```python
from build123d import *

# Parameters (mm, degrees)
SKETCH1_W                                       = 140
SKETCH1_H                                       = 220
BOSS_EXTRUDE1_DEPTH                             = 5
CUT_EXTRUDE1_DEPTH                              = 5
CHAMFER3_SIZE                                   = 15
F_4_0_4_DIAMETER_HOLE3_D                        = 4
F_4_0_4_DIAMETER_HOLE3_DEPTH                    = 5
F_4_0_4_DIAMETER_HOLE3_TIP                      = 1.201721238
CSK_FOR_M3_FLAT_HEAD_MACHINE_SCREW4_D           = 3.4
CSK_FOR_M3_FLAT_HEAD_MACHINE_SCREW4_DEPTH       = 5
CSK_FOR_M3_FLAT_HEAD_MACHINE_SCREW4_CSINK_D     = 6.3
CSK_FOR_M3_FLAT_HEAD_MACHINE_SCREW4_CSINK_ANGLE = 90
CSK_FOR_M3_FLAT_HEAD_MACHINE_SCREW4_TIP         = 1.021463052
SKETCH18_W                                      = 81.237331022
SKETCH18_H                                      = 9.628563132
CUT_EXTRUDE2_DEPTH                              = 5
CUT_EXTRUDE8_DEPTH                              = 10
SKETCH35_W                                      = 65
SKETCH35_H                                      = 45
CUT_EXTRUDE9_DEPTH                              = 131.479883507
FILLET1_R                                       = 2
CUT_EXTRUDE10_DEPTH                             = 131.479883507
SKETCH38_W                                      = 36
SKETCH38_H                                      = 20
CUT_EXTRUDE14_DEPTH                             = 131.479883507
SKETCH39_R                                      = 7
CUT_EXTRUDE15_DEPTH                             = 131.479883507
CSK_FOR_M3_FLAT_HEAD_MACHINE_SCREW3_D           = 3.4
CSK_FOR_M3_FLAT_HEAD_MACHINE_SCREW3_DEPTH       = 10
CSK_FOR_M3_FLAT_HEAD_MACHINE_SCREW3_CSINK_D     = 6.3
CSK_FOR_M3_FLAT_HEAD_MACHINE_SCREW3_CSINK_ANGLE = 90
CSK_FOR_M3_FLAT_HEAD_MACHINE_SCREW3_TIP         = 1.021463052
BOSS_EXTRUDE2_START                             = -3
SKETCH42_R                                      = 7
SKETCH42_R_2                                    = 4.25
BOSS_EXTRUDE2_DEPTH                             = 3
BOSS_EXTRUDE3_START                             = 8
SKETCH43_R                                      = 9
SKETCH43_R_2                                    = 7
BOSS_EXTRUDE3_DEPTH                             = 8
F_4_0MM_DOWEL_HOLE1_AT_2_COUNT                  = 2
F_4_0MM_DOWEL_HOLE1_AT_2_PITCH                  = 108.54146673
CUT_EXTRUDE16_DEPTH                             = 2
BOSS_EXTRUDE4_DEPTH                             = 5
CSK_FOR_M3_FLAT_HEAD_MACHINE_SCREW2_D           = 3.4
CSK_FOR_M3_FLAT_HEAD_MACHINE_SCREW2_DEPTH       = 5
CSK_FOR_M3_FLAT_HEAD_MACHINE_SCREW2_CSINK_D     = 6.3
CSK_FOR_M3_FLAT_HEAD_MACHINE_SCREW2_CSINK_ANGLE = 90
CSK_FOR_M3_FLAT_HEAD_MACHINE_SCREW2_TIP         = 1.021463052
FILLET3_R                                       = 2


with BuildPart() as part:
    # Sketch1 → Boss-Extrude1 (new body)
    with BuildSketch(Plane(origin=(0, 0, 0), x_dir=(1, 0, 0), z_dir=(0, 1, 0))):
        Rectangle(SKETCH1_W, SKETCH1_H)
    extrude(amount=BOSS_EXTRUDE1_DEPTH)

    # Sketch8 → Cut-Extrude1 (cut)
    with BuildSketch(Plane(origin=(0, 5, 0), x_dir=(1, 0, 0), z_dir=(0, 1, 0))):
        Polygon((-70, 110), (-32.5, 110), (-32.5, 44.951905284), (-70, -20), align=None)
        Polygon((70, 110), (70, -20), (32.5, 44.951905284), (32.5, 110), align=None)
    extrude(amount=-CUT_EXTRUDE1_DEPTH, mode=Mode.SUBTRACT)

    # Chamfer3
    chamfer3_edges = [part.edges().sort_by_distance(p)[0] for p in [
        (70, 2.5, 110),
        (-70, 2.5, 110),
    ]]
    chamfer(chamfer3_edges, length=CHAMFER3_SIZE)

    # Ø4.0 (4) Diameter Hole3
    with Locations(Plane(origin=(0, 5, 0), x_dir=(1, 0, 0), z_dir=(0, 1, 0))):
        with Locations((-27, 78), (-27, 63), (-60.732233047, -90.125631329), (-50.125631329, -100.732233047), (50.125631329, -100.732233047), (60.732233047, -90.125631329), (27, 63), (27, 78)):
            Hole(F_4_0_4_DIAMETER_HOLE3_D / 2, depth=F_4_0_4_DIAMETER_HOLE3_DEPTH)
            with Locations((0, 0, -(F_4_0_4_DIAMETER_HOLE3_DEPTH + F_4_0_4_DIAMETER_HOLE3_TIP / 2))):  # 118° drill point
                Cone(0, F_4_0_4_DIAMETER_HOLE3_D / 2, F_4_0_4_DIAMETER_HOLE3_TIP, mode=Mode.SUBTRACT)

    # CSK for M3 Flat Head Machine Screw4
    with Locations(Plane.XZ):
        with Locations((37.5, -25), (-37.5, -25), (-25, -100), (25, -100)):
            CounterSinkHole(CSK_FOR_M3_FLAT_HEAD_MACHINE_SCREW4_D / 2, CSK_FOR_M3_FLAT_HEAD_MACHINE_SCREW4_CSINK_D / 2, depth=CSK_FOR_M3_FLAT_HEAD_MACHINE_SCREW4_DEPTH, counter_sink_angle=CSK_FOR_M3_FLAT_HEAD_MACHINE_SCREW4_CSINK_ANGLE)
            with Locations((0, 0, -(CSK_FOR_M3_FLAT_HEAD_MACHINE_SCREW4_DEPTH + CSK_FOR_M3_FLAT_HEAD_MACHINE_SCREW4_TIP / 2))):  # 118° drill point
                Cone(0, CSK_FOR_M3_FLAT_HEAD_MACHINE_SCREW4_D / 2, CSK_FOR_M3_FLAT_HEAD_MACHINE_SCREW4_TIP, mode=Mode.SUBTRACT)

    # Sketch18 → Cut-Extrude2 (cut)
    with BuildSketch(Plane(origin=(0, 5, 0), x_dir=(1, 0, 0), z_dir=(0, 1, 0))):
        with Locations((-5.815131093, 109.814281566)):
            Rectangle(SKETCH18_W, SKETCH18_H)
    extrude(amount=-CUT_EXTRUDE2_DEPTH, mode=Mode.SUBTRACT)

    # Sketch34 → Cut-Extrude8 (cut)
    with BuildSketch(Plane(origin=(0, 5, 0), x_dir=(1, 0, 0), z_dir=(0, 1, 0))):
        Polygon((-70, -20), (-60, -2.679491924), (-60, -72.679491924), (-70, -90), align=None)
        Polygon((70, -90), (70, -20), (60, -2.679491924), (60, -72.679491924), align=None)
    extrude(amount=-CUT_EXTRUDE8_DEPTH, mode=Mode.SUBTRACT)

    # Sketch35 → Cut-Extrude9 (cut, through all)
    with BuildSketch(Plane(origin=(0, 5, 0), x_dir=(1, 0, 0), z_dir=(0, 1, 0))):
        with Locations((2, -36)):
            Rectangle(SKETCH35_W, SKETCH35_H)
    extrude(amount=-CUT_EXTRUDE9_DEPTH, mode=Mode.SUBTRACT)

    # Fillet1
    fillet1_edges = [part.edges().sort_by_distance(p)[0] for p in [
        (34.5, 2.5, 13.5),
        (34.5, 2.5, 58.5),
        (-30.5, 2.5, 58.5),
        (-30.5, 2.5, 13.5),
    ]]
    fillet(fillet1_edges, radius=FILLET1_R)

    # Sketch36 → Cut-Extrude10 (cut, through all)
    with BuildSketch(Plane(origin=(0, 5, 0), x_dir=(1, 0, 0), z_dir=(0, 1, 0))):
        Polygon((-47.5, -110), (-37.5, -100), (37.5, -100), (47.5, -110), align=None)
    extrude(amount=-CUT_EXTRUDE10_DEPTH, mode=Mode.SUBTRACT)

    # Sketch38 → Cut-Extrude14 (cut, through all)
    with BuildSketch(Plane.XZ):
        with Locations((0, -95)):
            Rectangle(SKETCH38_W, SKETCH38_H)
    extrude(amount=-CUT_EXTRUDE14_DEPTH, mode=Mode.SUBTRACT)

    # Sketch39 → Cut-Extrude15 (cut, through all)
    with BuildSketch(Plane.XZ):
        with Locations(Location((-47.5, 30, 0), (0, 0, 270))):
            Circle(SKETCH39_R)
        with Locations(Location((47.5, 30, 0), (0, 0, 90))):
            Circle(SKETCH39_R)
    extrude(amount=-CUT_EXTRUDE15_DEPTH, mode=Mode.SUBTRACT)

    # CSK for M3 Flat Head Machine Screw3
    with Locations(Plane(origin=(0, 0, 0), x_dir=(-1, 0, 0), z_dir=(0, -1, 0))):
        with Locations((-58, -82), (58, -82)):
            CounterSinkHole(CSK_FOR_M3_FLAT_HEAD_MACHINE_SCREW3_D / 2, CSK_FOR_M3_FLAT_HEAD_MACHINE_SCREW3_CSINK_D / 2, depth=CSK_FOR_M3_FLAT_HEAD_MACHINE_SCREW3_DEPTH, counter_sink_angle=CSK_FOR_M3_FLAT_HEAD_MACHINE_SCREW3_CSINK_ANGLE)
            with Locations((0, 0, -(CSK_FOR_M3_FLAT_HEAD_MACHINE_SCREW3_DEPTH + CSK_FOR_M3_FLAT_HEAD_MACHINE_SCREW3_TIP / 2))):  # 118° drill point
                Cone(0, CSK_FOR_M3_FLAT_HEAD_MACHINE_SCREW3_D / 2, CSK_FOR_M3_FLAT_HEAD_MACHINE_SCREW3_TIP, mode=Mode.SUBTRACT)

    # Sketch42 → Boss-Extrude2 (add)
    # profile 1 of 2: a face of its own
    with BuildSketch(Plane(origin=(0, 5, 0), x_dir=(1, 0, 0), z_dir=(0, 1, 0)).offset(BOSS_EXTRUDE2_START)):
        with Locations(Location((-47.5, -30, 0), (0, 0, 90))):
            Circle(SKETCH42_R)
        with Locations(Location((-47.5, -30, 0), (0, 0, 270))):
            Circle(SKETCH42_R_2, mode=Mode.SUBTRACT)
    # profile 2 of 2: a face of its own
    with BuildSketch(Plane(origin=(0, 5, 0), x_dir=(1, 0, 0), z_dir=(0, 1, 0)).offset(BOSS_EXTRUDE2_START)):
        with Locations(Location((47.5, -30, 0), (0, 0, 90))):
            Circle(SKETCH42_R)
        with Locations(Location((47.5, -30, 0), (0, 0, 90))):
            Circle(SKETCH42_R_2, mode=Mode.SUBTRACT)
    extrude(amount=BOSS_EXTRUDE2_DEPTH)

    # Sketch43 → Boss-Extrude3 (add)
    # profile 1 of 2: a face of its own
    with BuildSketch(Plane.XZ.offset(BOSS_EXTRUDE3_START)):
        with Locations(Location((-47.5, 30, 0), (0, 0, 90))):
            Circle(SKETCH43_R)
        with Locations(Location((-47.5, 30, 0), (0, 0, 270))):
            Circle(SKETCH43_R_2, mode=Mode.SUBTRACT)
    # profile 2 of 2: a face of its own
    with BuildSketch(Plane.XZ.offset(BOSS_EXTRUDE3_START)):
        with Locations(Location((47.5, 30, 0), (0, 0, 90))):
            Circle(SKETCH43_R)
        with Locations(Location((47.5, 30, 0), (0, 0, 270))):
            Circle(SKETCH43_R_2, mode=Mode.SUBTRACT)
    extrude(amount=-BOSS_EXTRUDE3_DEPTH)

    # Sketch46 → Ø4.0mm Dowel Hole1 (revolve, cut)
    with BuildSketch(Plane(origin=(-54.5, 5, 54), x_dir=(0, 0, 1), z_dir=(1, 0, 0))):
        Polygon((0, 0), (0, 6.201721238), (2, 5), (2, 0), align=None)
    f_4_0mm_dowel_hole1 = revolve(axis=Axis((-54.5, 11.35, 54), (0, -1, 0)), mode=Mode.SUBTRACT)

    # Ø4.0mm Dowel Hole1 at 2: Ø4.0mm Dowel Hole1 ×2
    with Locations(*[Vector(0.2533593918376833, 0, -0.9673722233802454) * (i * F_4_0MM_DOWEL_HOLE1_AT_2_PITCH) for i in range(1, F_4_0MM_DOWEL_HOLE1_AT_2_COUNT)]):
        add(f_4_0mm_dowel_hole1, mode=Mode.SUBTRACT)

    # Mirror1: Ø4.0mm Dowel Hole1 across plane
    add(f_4_0mm_dowel_hole1.mirror(Plane(origin=(0, 0, 0), x_dir=(0, 0, 1), z_dir=(1, 0, 0))), mode=Mode.SUBTRACT)

    # Mirror1 copy 1 sketch → Mirror1 copy 1 (revolve, cut)
    with BuildSketch(Plane(origin=(27, 5, -51), x_dir=(0, 0, 1), z_dir=(-1, 0, 0))):
        Polygon((0, 0), (0, -6.201721238), (2, -5), (2, 0), align=None)
    revolve(axis=Axis((27, 11.35, -51), (0, 1, 0)), mode=Mode.SUBTRACT)

    # Sketch47 → Cut-Extrude16 (cut)
    with BuildSketch(Plane(origin=(0, 5, 0), x_dir=(1, 0, 0), z_dir=(0, 1, 0))):
        Polygon((29.8, 49.383419246), (29.8, 52.616580754), (27, 54.233161507), (24.2, 52.616580754), (24.2, 49.383419246), (27, 47.766838493), align=None)
        Polygon((57.3, -55.616580754), (57.3, -52.383419246), (54.5, -50.766838493), (51.7, -52.383419246), (51.7, -55.616580754), (54.5, -57.233161507), align=None)
        Polygon((-54.5, -57.233161507), (-57.3, -55.616580754), (-57.3, -52.383419246), (-54.5, -50.766838493), (-51.7, -52.383419246), (-51.7, -55.616580754), align=None)
        Polygon((-27, 47.766838493), (-29.8, 49.383419246), (-29.8, 52.616580754), (-27, 54.233161507), (-24.2, 52.616580754), (-24.2, 49.383419246), align=None)
    extrude(amount=-CUT_EXTRUDE16_DEPTH, mode=Mode.SUBTRACT)

    # Sketch48 → Boss-Extrude4 (add)
    with BuildSketch(Plane(origin=(0, 5, 0), x_dir=(1, 0, 0), z_dir=(0, 1, 0))):
        Polygon((32.5, 58), (32.5, 83), (37.5, 78), (37.5, 63), align=None)
        Polygon((-32.5, 58), (-37.5, 63), (-37.5, 78), (-32.5, 83), align=None)
    extrude(amount=-BOSS_EXTRUDE4_DEPTH)

    # CSK for M3 Flat Head Machine Screw2
    with Locations(Plane(origin=(0, 0, 0), x_dir=(-1, 0, 0), z_dir=(0, -1, 0))):
        with Locations((27, 63), (27, 78), (-27, 78), (-27, 63), (60.732233047, -90.125631329), (50.125631329, -100.732233047), (-50.125631329, -100.732233047), (-60.732233047, -90.125631329)):
            CounterSinkHole(CSK_FOR_M3_FLAT_HEAD_MACHINE_SCREW2_D / 2, CSK_FOR_M3_FLAT_HEAD_MACHINE_SCREW2_CSINK_D / 2, depth=CSK_FOR_M3_FLAT_HEAD_MACHINE_SCREW2_DEPTH, counter_sink_angle=CSK_FOR_M3_FLAT_HEAD_MACHINE_SCREW2_CSINK_ANGLE)
            with Locations((0, 0, -(CSK_FOR_M3_FLAT_HEAD_MACHINE_SCREW2_DEPTH + CSK_FOR_M3_FLAT_HEAD_MACHINE_SCREW2_TIP / 2))):  # 118° drill point
                Cone(0, CSK_FOR_M3_FLAT_HEAD_MACHINE_SCREW2_D / 2, CSK_FOR_M3_FLAT_HEAD_MACHINE_SCREW2_TIP, mode=Mode.SUBTRACT)

    # Fillet3
    fillet3_edges = [part.edges().sort_by_distance(p)[0] for p in [
        (-32.5, 2.5, -105),
        (32.5, 2.5, -105),
        (-60, 2.5, 2.679491924),
        (60, 2.5, 2.679491924),
        (-60, 2.5, 72.679491924),
        (-70, 2.5, 90),
        (70, 2.5, 90),
        (60, 2.5, 72.679491924),
        (-32.5, 2.5, -44.951905284),
        (47.5, 2.5, 110),
        (-47.5, 2.5, 110),
        (-37.5, 2.5, 100),
        (37.5, 2.5, 100),
        (18, 2.5, -105),
        (-18, 2.5, -105),
        (-18, 2.5, -85),
        (18, 2.5, -85),
        (32.5, 2.5, -44.951905284),
        (70, 2.5, 95),
        (-55, 2.5, 110),
        (55, 2.5, 110),
        (-70, 2.5, 95),
    ]]
    fillet(fillet3_edges, radius=FILLET3_R)


solid = part.part
```
CAD build for the part. Positions are in the model's coordinates, mm. A direction names the side the tool comes from. Round coordinates to 2 decimals unless told otherwise and drop trailing zeros. Order: outer loops, then holes, each group sorted by start corner. A loop starts at its lowest first (then second) coordinate and runs counter-clockwise, first axis right, second up.
Q1. Drop flat-ended pins along their axis: pin 1 (6.5 mm diameter, centred on x = -27, z = -78, fed in from +Y); pin 2 (1.5 mm diameter, centred on x = -50.5, y = 1, fed in from -Z); pin 3 (5.5 mm diameter, centred on y = 2.5, z = 47.5, fed in from +X); pin 4 (5 mm diameter, centred on x = -33.5, y = 3, fed in from -Z). Give the stop position or say it passes through.
Q2. Slice it at B-B (z = -11.5). Write the cut outline in (x, y).
Q3. Wall check: L1, parallel to X at y = -1, z = 30; L2, parallel to X at y = 3.5, z = -100; L3, parallel to X at y = 1.55, z = -51. Give the ranges that are in metal, low to high.
Q4. Which spindle directions (+Z, -Z, +X, -X, +Y, -Y) get a long thin tool onto all of the face, cutting with end or side? Do faces 4 (the flat face through (-1, 3, 100)), 5 (the flat face through (-35, 2.5, -60.5)), 6 (the flat face through (34.5, 3, 36)), 7 (the cylindrical face through (-41.598, -3.07, 26.237)). Say none if no direction does.
Q5. Two-plate mould, pull along Z, no slides. Class faces 1 (the flat face through (32.5, 3, -52)), 2 (the flat face through (-25, 3, -105)), 3 (the flat face through (-37.5, 3, -70)): pulls with the +Z half, pulls with the -Z half, needs draft (parallel to the pull), parting line crosses it, or undercut.
Q6. Slice it at A-A (y = -2.25). Write the cut outline in (x, z).
Results below:
1. pin 1: stops at y = 5
1. pin 2: stops at z = -15.07
1. pin 3: stops at x = 60
1. pin 4: stops at z = -104.94
2. outline: (-51.81, 0) - (51.81, 0) - (51.81, 5) - (-51.81, 5) - close
3. L1: x = -56.5 to -54.5, -40.5 to -38.5, 38.5 to 40.5, 54.5 to 56.5
3. L2: x = -32.5 to -26.7, -23.3 to -18, 18 to 23.3, 26.7 to 32.5
3. L3: x = -32.5 to -29, -25 to 25, 29 to 32.5
4. face 4: +Z, +Y, -Y
4. face 5: -X, +Y, -Y
4. face 6: +Y, -Y
4. face 7: -Y
5. face 1: undercut
5. face 2: pulls with the -Z half
5. face 3: needs draft
6. outline: circle Ø18 at (-47.5, 30); circle Ø18 at (47.5, 30); hole circle Ø14 at (-47.5, 30); hole circle Ø14 at (47.5, 30)
